Can you work these out from the drawing? Everything is in mm from the part's minimum corner. A direction names the side the tool comes from. Give positions to 0.01 mm unless a question says otherwise; leave off trailing zeros. Write each loop counter-clockwise with the first axis right and the second up, starting at its lowest first coordinate (ties: lowest second). Pieces come first, ordered by that corner, then holes. Notation, with made-up numbers: (-3, 32) - (27, 32) arc R23 cw to (27, 41) - close; hole circle Ø9 at (54.25, 53). An arc over 180 degrees is marked (long way). Write each question's results on one line, items separated by ' | '. Start each with the question number.
Item 1: Suppose I cut it at C-C on z = 6. List the corners of the cut face in (x, y) for me (1 decimal).
Item 2: Suppose I cut it at D-D on x = 41. List the corners of the cut face in (y, z) for me (1 decimal), then the cut area to 3 significant figures.
Item 3: Suppose I cut it at B-B on y = 71. List the corners of the cut face in (x, z) for me, then the cut area to 3 significant figures.
Item 4: Which directions (+Z, -Z, +X, -X, +Y, -Y) give clear straight access to the entire face, cutting with the end or side of a thin tool? Please do the marked faces 1, 2, 3, 4 and 5.
Item 5: Please list where these lines run through material, in increasing order: line 1 along X through (y, z) = (72, 49); line 2 along X through (y, z) = (27.5, 9); line 3 along X through (y, z) = (65, 94).
Item 6: We'd pull the mould along X, two halves only. Please class the marked faces 6, 7 and 8: +X half, -X half, draft (parallel to the pull), parting line (faces both ways), or undercut.
Item 7: Suppose I cut it at A-A on z = 50. List the corners of the cut face in (x, y) for me (1 decimal), then the cut area to 3 significant figures.
Item 8: Will these pins go through, and if not, where does the flat tip stop? P1, Ø12.5, axis at x = 178, y = 37, coming from the +Z side; P2, Ø6, axis at x = 146.5, z = 70.5, coming from the +Y side; P3, Ø8, axis at y = 69, z = 57, coming from the -X side; P4, Ø20, axis at x = 147, y = 30.5, coming from the +Z side.
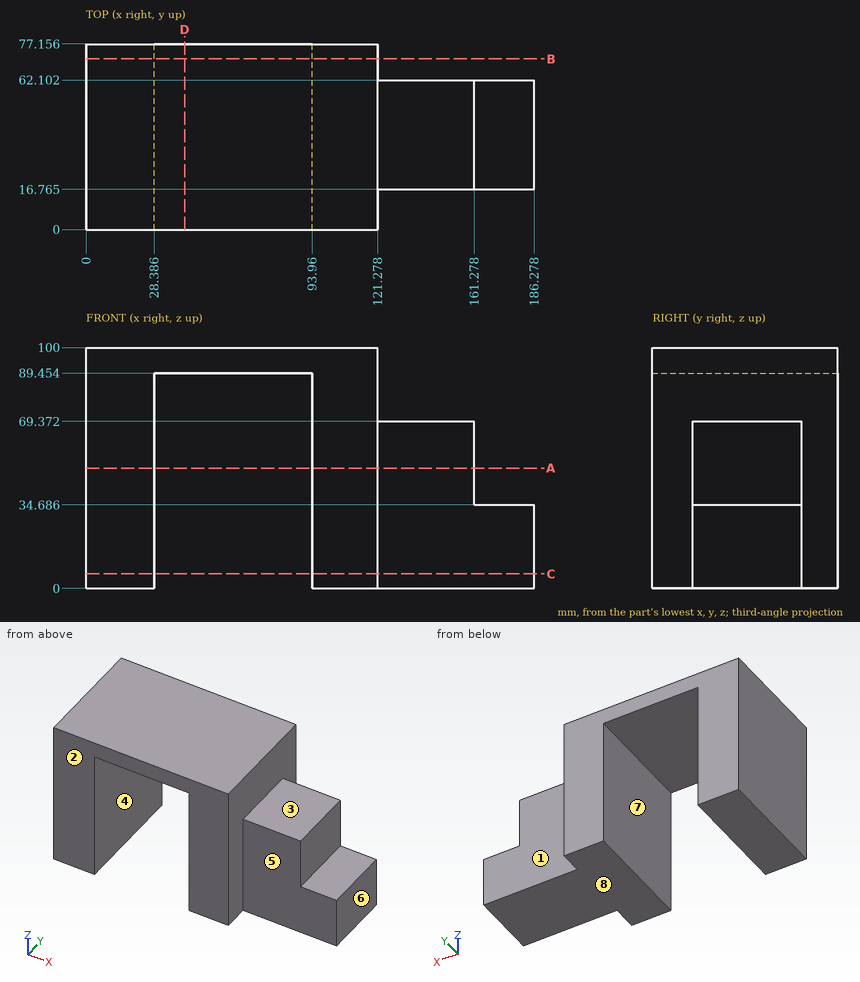
Checked values:
1) outline: (0, 0) - (28.4, 0) - (28.4, 77.2) - (0, 77.2) - close; (94, 0) - (121.3, 0) - (121.3, 16.8) - (186.3, 16.8) - (186.3, 62.1) - (121.3, 62.1) - (121.3, 77.2) - (94, 77.2) - close
2) outline: (0, 89.5) - (77.2, 89.5) - (77.2, 100) - (0, 100) - close | area: 814 mm^2
3) outline: (0, 0) - (28.39, 0) - (28.39, 89.45) - (93.96, 89.45) - (93.96, 0) - (121.28, 0) - (121.28, 100) - (0, 100) - close | area: 6,260 mm^2
4) face 1: +Z, -Z, +X, +Y | face 2: +Z, -Z, +X, -X, -Y | face 3: +Z, +X, +Y, -Y | face 4: -Z, +Y, -Y | face 5: +Z, -Z, +X, -Y
5) line 1: x = 0 to 28.39, 93.96 to 121.28 | line 2: x = 0 to 28.39, 93.96 to 186.28 | line 3: x = 0 to 121.28
6) face 6: +X half | face 7: undercut | face 8: draft
7) outline: (0, 0) - (28.4, 0) - (28.4, 77.2) - (0, 77.2) - close; (94, 0) - (121.3, 0) - (121.3, 16.8) - (161.3, 16.8) - (161.3, 62.1) - (121.3, 62.1) - (121.3, 77.2) - (94, 77.2) - close | area: 6,110 mm^2
8) P1: stops at z = 34.69 | P2: stops at y = 62.1 | P3: stops at x = 0 | P4: stops at z = 69.37
